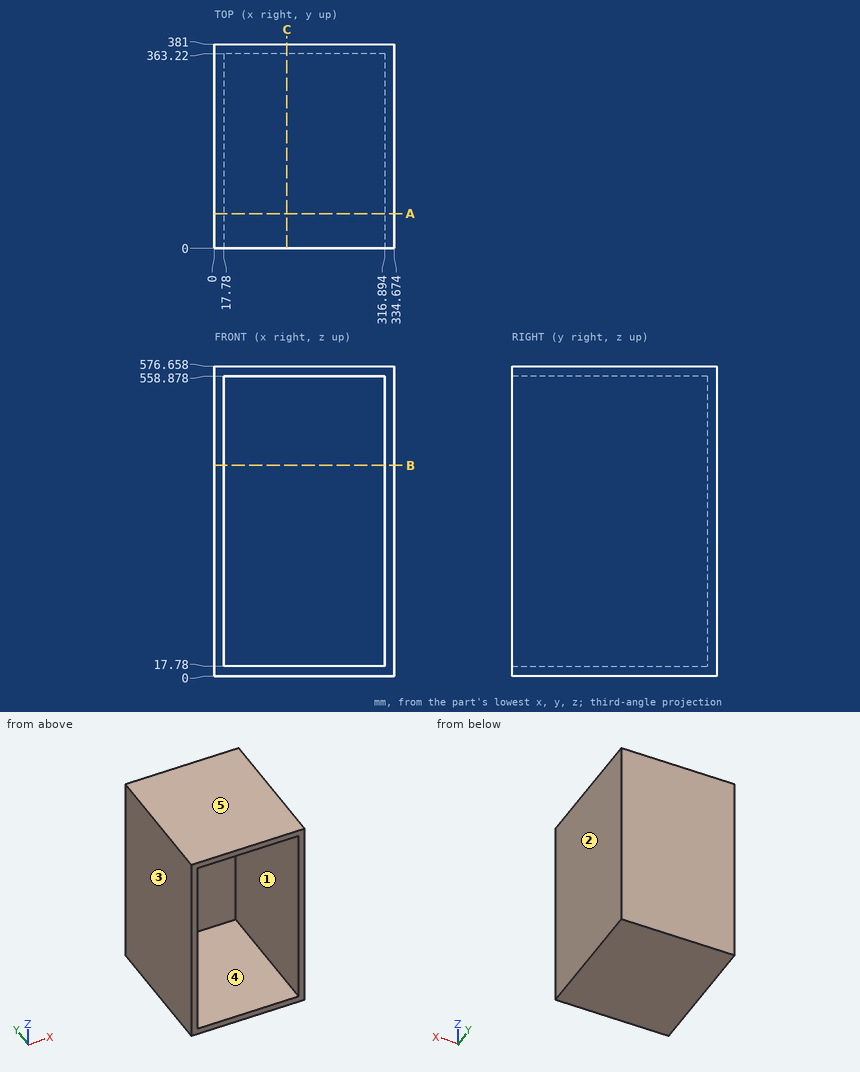
Geometry check sheet. Reference: drawing and pictorial views, mm from the part's lowest x, y, z. A direction names the side the tool comes from. Give positions to 0.01 mm unless a question says otherwise; leave off trailing zeros. Order: outer loops, then holes, each group sorted by start corner. A loop starts at its lowest first (then second) coordinate and runs counter-clockwise, first axis right, second up. Notation, with made-up numbers: M 18.5,25 L 69.5,25 A31 cw 69.5,55 Z; hole C 54,32 d1. An arc over 180 degrees is marked long. Answer as a JSON object with one key per item and string values. Group by question number.
1) Access from +Z, -Z, +X, -X, +Y, -Y to the whole of each face (thin tool, end or side, straight path). Record for the marked faces 1 and 2.
2) Mould release check, pull along X, two halves, no side actions. Record for the marked faces 3, 4 and 5: released by +X, released by -X, zero draft, split by the parting line, or undercut.
3) Cross-section at C-C (x = 135). Enter the section's corners in (y, z).
4) Cross-section at A-A (y = 65). Enter the section's corners in (x, z).
5) Cross-section at B-B (z = 392.5). Enter the section's corners in (x, y), then the cut area to 3 significant figures.
6) Scan lines: line 1 along Z through (x, y) = (174, 347.5); line 2 along X through (y, z) = (336, 388); line 3 along Y through (x, z) = (146, 306). Record each from-to range of solid material in increasing order. Write a range as [from, to].
Result sheet:
{
 "1": {"face 1": "-Y", "face 2": "+Z, -Z, +X, +Y, -Y"},
 "2": {"face 3": "released by -X", "face 4": "undercut", "face 5": "zero draft"},
 "3": {"outline": "M 0,0 L 381,0 L 381,576.66 L 0,576.66 L 0,558.88 L 363.22,558.88 L 363.22,17.78 L 0,17.78 Z"},
 "4": {"outline": "M 0,0 L 334.67,0 L 334.67,576.66 L 0,576.66 Z; hole M 17.78,17.78 L 316.89,17.78 L 316.89,558.88 L 17.78,558.88 Z"},
 "5": {"outline": "M 0,0 L 17.78,0 L 17.78,363.22 L 316.89,363.22 L 316.89,0 L 334.67,0 L 334.67,381 L 0,381 Z", "area": "18,900 mm2"},
 "6": {"line 1": "z = [0, 17.78], [558.88, 576.66]", "line 2": "x = [0, 17.78], [316.89, 334.67]", "line 3": "y = [363.22, 381]"}
}
